from build123d import *

# Parameters (mm, degrees)
SKETCH_W   = 220
SKETCH_H   = 300
SKETCH_R   = 10
SKETCH_R_2 = 2.5
SKETCH_R_3 = 5.5
SKETCH_R_4 = 2
SKETCH_R_5 = 4.5
PAD_DEPTH  = 5


with BuildPart() as part:
    # Sketch → Pad (new body)
    with BuildSketch(Plane.XZ):
        Rectangle(SKETCH_W, SKETCH_H)
        with Locations((0, 88)):
            Circle(SKETCH_R, mode=Mode.SUBTRACT)
        with Locations((25.4, 88)):
            Circle(SKETCH_R_2, mode=Mode.SUBTRACT)
        with Locations((-25.4, 88)):
            Circle(SKETCH_R_2, mode=Mode.SUBTRACT)
        with Locations((85, 88)):
            Circle(SKETCH_R_3, mode=Mode.SUBTRACT)
        with Locations((-85, 88)):
            Circle(SKETCH_R_3, mode=Mode.SUBTRACT)
        with Locations((-85, -88)):
            Circle(SKETCH_R_3, mode=Mode.SUBTRACT)
        with Locations((85, -88)):
            Circle(SKETCH_R_3, mode=Mode.SUBTRACT)
        with Locations((-90, 130)):
            Circle(SKETCH_R_4, mode=Mode.SUBTRACT)
        with Locations((90, 130)):
            Circle(SKETCH_R_4, mode=Mode.SUBTRACT)
        with Locations((-90, -130)):
            Circle(SKETCH_R_4, mode=Mode.SUBTRACT)
        with Locations((90, -130)):
            Circle(SKETCH_R_4, mode=Mode.SUBTRACT)
        with Locations((0, 135)):
            Circle(SKETCH_R_2, mode=Mode.SUBTRACT)
        with Locations((0, -135)):
            Circle(SKETCH_R_2, mode=Mode.SUBTRACT)
        with Locations((90, 0)):
            Circle(SKETCH_R_2, mode=Mode.SUBTRACT)
        with Locations((-90, 0)):
            Circle(SKETCH_R_2, mode=Mode.SUBTRACT)
        with Locations((-90, -60)):
            Circle(SKETCH_R_2, mode=Mode.SUBTRACT)
        with Locations((-90, 60)):
            Circle(SKETCH_R_2, mode=Mode.SUBTRACT)
        with Locations((90, 60)):
            Circle(SKETCH_R_2, mode=Mode.SUBTRACT)
        with Locations((90, -60)):
            Circle(SKETCH_R_2, mode=Mode.SUBTRACT)
        with Locations((0, -88)):
            Circle(SKETCH_R_5, mode=Mode.SUBTRACT)
        with Locations((12.75, -75.25)):
            Circle(SKETCH_R_4, mode=Mode.SUBTRACT)
        with Locations((-12.75, -75.25)):
            Circle(SKETCH_R_4, mode=Mode.SUBTRACT)
        with Locations((-12.75, -100.75)):
            Circle(SKETCH_R_4, mode=Mode.SUBTRACT)
        with Locations((12.75, -100.75)):
            Circle(SKETCH_R_4, mode=Mode.SUBTRACT)
    extrude(amount=PAD_DEPTH)


solid = part.part
Work out the finished part from the listing and answer in its coordinate system (mm). Give positions to 0.01 mm unless a question says otherwise; leave off trailing zeros. Loops run counter-clockwise (first coordinate to the right, second up) from the corner with the lowest first, then second, coordinate; pieces in that order, holes last. Notation, with made-up numbers: (-20, -6.5) -> (35, -6.5) arc R23 cw to (35, 5.5) -> close; hole circle Ø4 at (57, -0.75). An arc over 180 degrees is marked (long way). Use a Markdown table: item, result. Add a question column.
1) The part is cut by section A-A, the plane z = -88. Determine the outline of the cut face in (x, y).
2) The part is cut by section B-B, the plane y = -2.55. Count the separate pieces of the cut face and the enclosed holes in it, plus the area to 3 significant figures.
3) Each of these flat-tipped pins is pushed along its axis until it touches: P1, Ø3.5, axis at x = 90, z = -130, coming from the +Y side; P2, Ø6.5, axis at x = 90, z = 60, coming from the -Y side. Where does it stop, or does it pass through?
4) Consider line 1 along Z through (x, y) = (0, -1.1); line 2 along X through (y, z) = (-3.4, -87.5); line 3 along Z through (x, y) = (12.75, -2.1). Determine where each line is inside the solid, lowest interval first.
5) For a pull along Z with two mould halves and no side action, classify faces 1 (the flat face through (-2, -5, 2)), 2 (the cylindrical face through (-1.302, -2.465, 97.915)), 3 (the cylindrical face through (80.95, -2.46, -84.28)) as +Z half, -Z half, draft (parallel to the pull), parting line (faces both ways), or undercut.
Reported:
| question | item | result |
|---|---|---|
| 1 | outline | (-110, -5) -> (-90.5, -5) -> (-90.5, 0) -> (-110, 0) -> close; (-79.5, -5) -> (-4.5, -5) -> (-4.5, 0) -> (-79.5, 0) -> close; (4.5, -5) -> (79.5, -5) -> (79.5, 0) -> (4.5, 0) -> close; (90.5, -5) -> (110, -5) -> (110, 0) -> (90.5, 0) -> close |
| 2 | separate pieces | 1 |
| 2 | enclosed holes | 24 |
| 2 | area | 64,900 mm^2 |
| 3 | P1 | passes through |
| 3 | P2 | stops at y = -5 |
| 4 | line 1 | z = -150 to -137.5, -132.5 to -92.5, -83.5 to 78, 98 to 132.5, 137.5 to 150 |
| 4 | line 2 | x = -110 to -90.48, -79.52 to -4.47, 4.47 to 79.52, 90.48 to 110 |
| 4 | line 3 | z = -150 to -102.75, -98.75 to -77.25, -73.25 to 150 |
| 5 | face 1 | draft |
| 5 | face 2 | undercut |
| 5 | face 3 | undercut |
